```python
from build123d import *

# Parameters (mm, degrees)
SKETCH1_W                                    = 165.1
SKETCH1_H                                    = 165.1
SKETCH1_R                                    = 13.096875
SKETCH1_R_2                                  = 1.5875
BOSS_EXTRUDE1_DEPTH                          = 6.35
SKETCH3_R                                    = 15.875
CUT_EXTRUDE1_DEPTH                           = 4.7625
CSK_FOR_1_4_FLAT_HEAD_SOCKET_CAP_SCR_2_COUNT = 2
CSK_FOR_1_4_FLAT_HEAD_SOCKET_CAP_SCR_2_PITCH = 81.28
CSK_FOR_1_4_FLAT_HEAD_SOCKET_CAP_SCR_3_COUNT = 2
CSK_FOR_1_4_FLAT_HEAD_SOCKET_CAP_SCR_3_PITCH = 69.342
FILLET1_R                                    = 6.35
F_10_CLEARANCE_HOLE1_D                       = 5.1054
F_1_4_20_TAPPED_HOLE1_D                      = 5.1054
F_1_4_20_TAPPED_HOLE1_DEPTH                  = 16.002
F_1_4_20_TAPPED_HOLE1_TIP                    = 1.533816902
F_10_CLEARANCE_HOLE2_D                       = 5.1054
SKETCH16_R                                   = 8.9027
SKETCH16_R_2                                 = 19.446875
SKETCH16_R_3                                 = 7.332969894
SKETCH16_R_4                                 = 9.7282
CUT_EXTRUDE2_DEPTH                           = 3.175
FILLET2_R                                    = 3.175


with BuildPart() as part:
    # Sketch1 → Boss-Extrude1 (new body)
    with BuildSketch(Plane(origin=(0, 0, 0), x_dir=(1, 0, 0), z_dir=(0, 1, 0))):
        Rectangle(SKETCH1_W, SKETCH1_H)
        with Locations((-19.05, -12.7)):
            Circle(SKETCH1_R, mode=Mode.SUBTRACT)
        with Locations((23.8125, -12.7)):
            Circle(SKETCH1_R_2, mode=Mode.SUBTRACT)
    extrude(amount=BOSS_EXTRUDE1_DEPTH)

    # Sketch3 → Cut-Extrude1 (cut)
    with BuildSketch(Plane.XZ.offset(-6.35)):
        with Locations((-19.05, 12.7)):
            Circle(SKETCH3_R)
    extrude(amount=CUT_EXTRUDE1_DEPTH, mode=Mode.SUBTRACT)

    # Sketch8 → CSK for 1/4 Flat Head Socket Cap Screw1 (revolve, cut)
    with BuildSketch(Plane(origin=(-61.255776472, 6.35, 18.990629251), x_dir=(0, 0, 1), z_dir=(1, 0, 0))):
        Polygon((0, 0), (0, 6.35), (3.3782, 6.35), (3.3782, 3.871564875), (6.7437, 0), align=None)
    csk_for_1_4_flat_head_socket_cap_screw1 = revolve(axis=Axis((-61.255776472, 12.7, 18.990629251), (0, -1, 0)), mode=Mode.SUBTRACT)

    # CSK for 1_4 Flat Head Socket Cap Scr 2: CSK for 1/4 Flat Head Socket Cap Screw1 ×2
    with Locations(*[Vector(0.938375852, 0, -0.345616493) * (i * CSK_FOR_1_4_FLAT_HEAD_SOCKET_CAP_SCR_2_PITCH) for i in range(1, CSK_FOR_1_4_FLAT_HEAD_SOCKET_CAP_SCR_2_COUNT)]):
        add(csk_for_1_4_flat_head_socket_cap_screw1, mode=Mode.SUBTRACT)

    # CSK for 1_4 Flat Head Socket Cap Scr 3: CSK for 1/4 Flat Head Socket Cap Screw1 ×2
    with Locations(*[Vector(0.846756316, 0, 0.531980959) * (i * CSK_FOR_1_4_FLAT_HEAD_SOCKET_CAP_SCR_3_PITCH) for i in range(1, CSK_FOR_1_4_FLAT_HEAD_SOCKET_CAP_SCR_3_COUNT)]):
        add(csk_for_1_4_flat_head_socket_cap_screw1, mode=Mode.SUBTRACT)

    # Fillet1
    fillet1_edges = [part.edges().sort_by_distance(p)[0] for p in [
        (-82.55, 3.175, -82.55),
        (82.55, 3.175, -82.55),
        (82.55, 3.175, 82.55),
        (-82.55, 3.175, 82.55),
    ]]
    fillet(fillet1_edges, radius=FILLET1_R)

    # #10 Clearance Hole1 (through all)
    with Locations(Plane(origin=(0, 6.35, 0), x_dir=(1, 0, 0), z_dir=(0, 1, 0))):
        with Locations((-76.2, -76.2), (-76.2, 76.2), (76.2, 76.2), (76.2, -76.2), (0, 76.2), (0, -76.2), (-76.2, 0), (76.2, 0)):
            Hole(F_10_CLEARANCE_HOLE1_D / 2)

    # 1/4-20 Tapped Hole1
    with Locations(Plane(origin=(0, 6.35, 0), x_dir=(1, 0, 0), z_dir=(0, 1, 0))):
        with Locations((23.8125, -12.7), (-49.358364409, -43.008364409), (-19.05, 30.1625), (-19.05, -12.7)):
            Hole(F_1_4_20_TAPPED_HOLE1_D / 2, depth=F_1_4_20_TAPPED_HOLE1_DEPTH)
            with Locations((0, 0, -(F_1_4_20_TAPPED_HOLE1_DEPTH + F_1_4_20_TAPPED_HOLE1_TIP / 2))):  # 118° drill point
                Cone(0, F_1_4_20_TAPPED_HOLE1_D / 2, F_1_4_20_TAPPED_HOLE1_TIP, mode=Mode.SUBTRACT)

    # #10 Clearance Hole2 (through all)
    with Locations(Plane(origin=(0, 6.35, 0), x_dir=(1, 0, 0), z_dir=(0, 1, 0))):
        with Locations((23.8125, 30.1625), (4.7625, 30.1625)):
            Hole(F_10_CLEARANCE_HOLE2_D / 2)

    # Sketch16 → Cut-Extrude2 (cut)
    with BuildSketch(Plane.XZ):
        with BuildLine():
            Line((-69.85, -69.85), (69.85, -69.85))
            Line((69.85, -69.85), (69.85, 69.85))
            Line((69.85, 69.85), (-69.85, 69.85))
            Line((-69.85, 69.85), (-69.85, 23.548830343))
            ThreePointArc((-69.85, 23.548830343), (-51.527576472, 18.990629251), (-69.85, 14.432428159))
            Line((-69.85, 14.432428159), (-69.85, -69.85))
        make_face()
        with Locations((-19.05, -30.1625)):
            Circle(SKETCH16_R, mode=Mode.SUBTRACT)
        with BuildLine():
            ThreePointArc((26.701812238, 4.279195877), (25.431817694, 3.945808004), (24.126599504, 3.802842657))
            ThreePointArc((24.126599504, 3.802842657), (21.821072601, 1.296842431), (21.77826487, -2.108103813))
            ThreePointArc((21.77826487, -2.108103813), (22.726285123, -3.169779078), (23.509240054, -4.358424671))
            ThreePointArc((23.509240054, -4.358424671), (24.7390513, -9.398953448), (23.203012358, -14.354753124))
            ThreePointArc((23.203012358, -14.354753124), (22.778841422, -18.668760314), (26.026775263, -21.539562429))
            ThreePointArc((26.026775263, -21.539562429), (31.576627013, -34.518690884), (17.607086431, -36.546143923))
            ThreePointArc((17.607086431, -36.546143923), (14.2875, -35.198574694), (10.967913569, -36.546143923))
            ThreePointArc((10.967913569, -36.546143923), (-3.202448667, -34.139642192), (3.388256312, -21.366505367))
            ThreePointArc((3.388256312, -21.366505367), (6.975124047, -18.66147581), (6.716089287, -14.176422182))
            ThreePointArc((6.716089287, -14.176422182), (6.098886497, -5.210907818), (13.090804558, 0.434840043))
            ThreePointArc((13.090804558, 0.434840043), (13.280061368, 0.471090255), (13.469999062, 0.503584721))
            ThreePointArc((13.469999062, 0.503584721), (16.805475765, 3.267308056), (16.522545733, 7.589752053))
            ThreePointArc((16.522545733, 7.589752053), (26.565926614, 21.166209847), (26.701812238, 4.279195877))
        make_face(mode=Mode.SUBTRACT)
        with Locations((-19.05, 12.7)):
            Circle(SKETCH16_R_2, mode=Mode.SUBTRACT)
        with Locations((-49.358364409, 43.008364409)):
            Circle(SKETCH16_R_3, mode=Mode.SUBTRACT)
        with Locations((-2.54, 55.879252935)):
            Circle(SKETCH16_R_4, mode=Mode.SUBTRACT)
    extrude(amount=-CUT_EXTRUDE2_DEPTH, mode=Mode.SUBTRACT)

    # Fillet2
    fillet2_edges = [part.edges().sort_by_distance(p)[0] for p in [
        (-69.85, 1.5875, 14.432428159),
        (-69.85, 1.5875, 23.548830343),
        (-69.85, 1.5875, 69.85),
        (69.85, 1.5875, 69.85),
        (69.85, 1.5875, -69.85),
        (-69.85, 1.5875, -69.85),
    ]]
    fillet(fillet2_edges, radius=FILLET2_R)


solid = part.part
```
Can you work these out from the model? Positions are in its coordinate system, mm. A direction names the side the tool comes from. Round coordinates to 2 decimals unless told otherwise and drop trailing zeros. Loops run counter-clockwise (first coordinate to the right, second up) from the corner with the lowest first, then second, coordinate; pieces in that order, holes last. Notation, with made-up numbers: (20, 65.25) -> (45, 65.25) arc R21 ccw to (45, 77.25) -> close; hole circle Ø7 at (7.25, -39.5). An arc over 180 degrees is marked (long way). One line per item, written item: value. Start each with the question number.
1. For faces 1 (the cylindrical face through (-80.74, 3.22, 80.64)), 2 (the cylindrical face through (-45.416, 1.565, 49.192)), which set-ups out of +Z, -Z, +X, -X, +Y, -Y let a thin tool reach every point of the face, with its end or its side?
2. For pin 1 (8 mm diameter, centred on x = -61, z = 38, fed in from -Y) (3 decimals), with a flat end and sliding along its axis, tell me the tip position at first contact or that it passes through.
3. If we section it at A-A, the plane x = -19.05: Give the number of separate pieces and of enclosed holes in the cut face, then the cut area to 3 significant figures.
4. If we section it at B-B, the plane z = -58.5: Write out the boundary of the cut face in (x, y) (3 decimals).
5. If we mould it in two halves opening along Z, with no side actions, what happens to faces 3 (the flat face through (-46, 0, 43)), 4 (the cylindrical face through (-32.134, 0.783, 12.124)), 5 (the cylindrical face through (80.64, 3.22, -80.74))? For each: pulls with the +Z half, pulls with the -Z half, needs draft (parallel to the pull), parting line crosses it, or undercut.
6. If I drill on probe 1 along X at (y, z) = (5.25, 76.2); probe 2 along Z at (x, y) = (29, 1.5), over which ranges is the centre line in solid material (lowest first)?
Calculated:
1. face 1: +Z, -X, +Y, -Y
1. face 2: -Y
2. pin 1: stops at y = 3.175
3. separate pieces: 3
3. enclosed holes: 0
3. area: 560 mm²
4. outline: (-82.55, 0) -> (-69.85, 0) -> (-69.85, 3.175) -> (69.85, 3.175) -> (69.85, 0) -> (82.55, 0) -> (82.55, 6.35) -> (-82.55, 6.35) -> close
5. face 3: needs draft
5. face 4: undercut
5. face 5: pulls with the -Z half
6. probe 1: x = -82.55 to -78.75, -73.65 to -2.55, 2.55 to 73.65, 78.75 to 82.55
6. probe 2: z = -82.55 to -69.85, -37.4 to -22.93, 5.46 to 19.94, 69.85 to 82.55
